Verification items for this drawing (mm, ordinates from the low corner). Round coordinates to 2 decimals unless told otherwise and drop trailing zeros. Order: outer loops, then holes, each group sorted by start corner. A loop starts at its lowest first (then second) coordinate and runs counter-clockwise, first axis right, second up. Notation, with made-up numbers: M 69,64.25 L 116,64.25 A30 cw 116,88.25 Z; hole C 71,-19.75 d9. An arc over 180 degrees is marked long. One line per item, written item: value. Start each with the question number.
(1) Cross-section at A-A, the plane x = 5.5. Enter the section's corners in (y, z), and give its area (3 significant figures).
(2) Cross-section at D-D, the plane z = 39.5. Enter the section's corners in (x, y) (1 decimal).
(3) Depth check by flat-ended pin: pin 1 Ø12 at (y, z) = (92.5, 25.5) entering from -X; pin 2 Ø2 at (x, z) = (21, 40.5) entering from -Y; pin 3 Ø2 at (x, z) = (18.5, 38) entering from +Y; pin 4 Ø6 at (x, y) = (12, 76.5) entering from +Z. Enter the tip coordinate at first touch or a pass-through.
(4) Thickness scan on L1, parallel to Y at x = 17, z = 16.5; L2, parallel to X at y = 171, z = 25.5 (1 decimal); L3, parallel to Y at x = 17.5, z = 5. Record the ranges inside material, lowest first.
(5) Cross-section at C-C, the plane y = 54. Enter the section's corners in (x, z) (1 decimal), and give its area (3 significant figures).
(6) Release check for a two-part mould opening along Y. For the marked faces 1, 2 and 3 record: released by +Y, released by -Y, zero draft, split by the parting line, or undercut.
(7) Cross-section at B-B, the plane z = 22.5. Enter the section's corners in (x, y) (1 decimal).
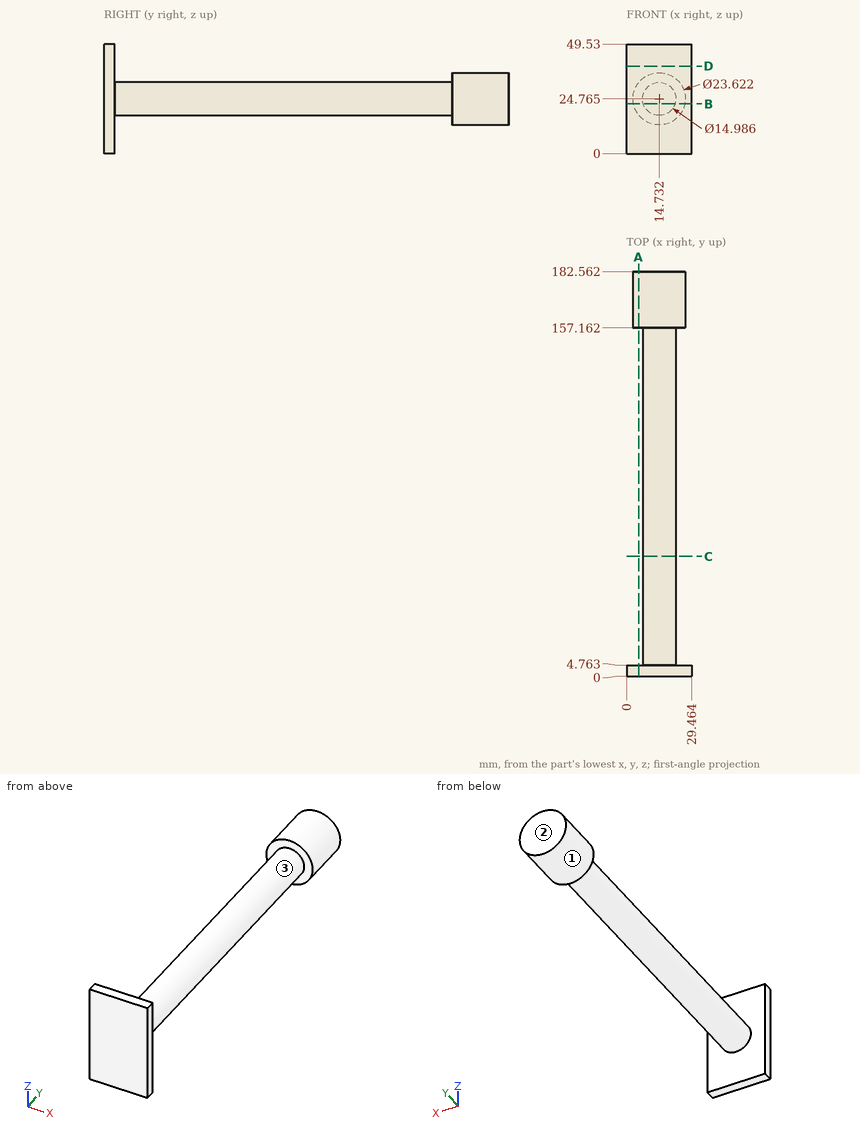
Values found:
1. outline: M 0,0 L 4.76,0 L 4.76,49.53 L 0,49.53 Z; M 157.16,17.4 L 182.56,17.4 L 182.56,32.13 L 157.16,32.13 Z
1. area: 610 mm^2
2. outline: M 0,0 L 29.5,0 L 29.5,4.8 L 0,4.8 Z
3. pin 1: x = 7.24
3. pin 2: y = 0
3. pin 3: y = 4.76
3. pin 4: z = 32.26
4. L1: 0 to 4.76, 157.16 to 182.56
4. L2: 2.9 to 26.5
4. L3: 0 to 4.76
5. outline: C 14.7,24.8 d15
5. area: 176 mm^2
6. face 1: zero draft
6. face 2: released by +Y
6. face 3: undercut
7. outline: M 0,0 L 29.5,0 L 29.5,4.8 L 21.9,4.8 L 21.9,157.2 L 26.3,157.2 L 26.3,182.6 L 3.1,182.6 L 3.1,157.2 L 7.6,157.2 L 7.6,4.8 L 0,4.8 Z
